CAD build for the part. Positions are in the model's coordinates, mm. A direction names the side the tool comes from. Coordinates: 2 decimals unless noted, no trailing zeros. Order: outer loops, then holes, each group sorted by start corner. A loop starts at its lowest first (then second) coordinate and runs counter-clockwise, first axis right, second up. Notation, with made-up numbers: M 43.25,23 L 91.25,23 A26 ccw 91.25,39 Z; hole C 48,-22.75 d10. An arc over 180 degrees is marked long. One line per item, written item: value.
Autodesk Inventor part; units mm, degrees
ref_plane "YZ Plane" through (0, 0, 0) normal (1, 0, 0) x (0, 1, 0)
ref_plane "XZ Plane" through (0, 0, 0) normal (0, 1, 0) x (-1, 0, 0)
ref_plane "XY Plane" through (0, 0, 0) normal (0, 0, 1) x (1, 0, 0)
sketch "Sketch1" plane through (0, 0, 0) normal (0, 0, 1) x (1, 0, 0)
  line L0 (0, 16.24) -> (0, -16.24) construction
  line L1 (-10, 0) -> (60, 0) construction
  line L2 (50, 11.6) -> (50, 9.6)
  line L3 (50, 9.6) -> (32, 9.6)
  line L4 (28, 11.6) -> (28, -9.6)
  line L5 (28, -9.6) -> (13, -9.6)
  line L6 (13, -9.6) -> (13, -11.6)
  line L7 (13, -11.6) -> (32, -11.6)
  line L8 (32, -11.6) -> (32, 9.6)
  line L9 (28, 11.6) -> (50, 11.6)
  point P0 (0, 0)
  dimension "d0" = 2
  dimension "d1" = 2
  dimension "d4" = 50
  dimension "d7" = 13
  dimension "d11" = 19.2
  dimension "d35" = 32
  dimension "d36" = 4
  dimension "d37" = 21.2
revolve "Revolution1" add sketch "Sketch1" angle 360 about axis through (0, 0, 0) along (0, -1, 0)
sketch "Sketch2" plane through (0, -9.6, 0) normal (0, -1, 0) x (1, 0, 0)
  line L0 (0, 70) -> (0, -70) construction
  line L1 (-70, 0) -> (70, 0) construction
  circle A0 centre (0, 0) radius 13 construction
  circle A1 centre (0, 0) radius 32 construction
  line L2 (15.5, -15.5) -> (-15.5, -15.5) construction
  line L3 (-15.5, -15.5) -> (-15.5, 15.5) construction
  line L4 (-15.5, 15.5) -> (15.5, 15.5) construction
  line L5 (15.5, 15.5) -> (15.5, -15.5) construction
  dimension "d14" = 31
  dimension "d15" = 31
hole "Hole1" at (15.5, -9.6, -15.5) at (-15.5, -9.6, -15.5) at (-15.5, -9.6, 15.5) at (15.5, -9.6, 15.5) direction (0, -1, 0) diameter 3.4 end through all countersink diameter 6.3 countersink angle 90
sketch "Sketch3" plane through (0, 11.6, 0) normal (0, 1, 0) x (1, 0, 0)
  line L0 (0, 70) -> (0, -70) construction
  line L1 (70, 0) -> (-70, 0) construction
  circle A0 centre (0, 0) radius 45 construction
  point P0 (0, 45)
  point P1 (-38.9711, 22.5)
  point P2 (-38.9711, -22.5)
  point P3 (0, -45)
  point P4 (38.9711, -22.5)
  point P5 (38.9711, 22.5)
  dimension "d23" = 90
  dimension "d26" = 360
hole "Hole2" at (0, 11.6, -45) at (-38.9711, 11.6, -22.5) at (-38.9711, 11.6, 22.5) at (0, 11.6, 45) at (38.9711, 11.6, 22.5) at (38.9711, 11.6, -22.5) direction (0, -1, 0) diameter 3.4 depth 2
fillet "Fillet1" radius 5 1 edges at (-32, 9.6, 0)
sketch "Sketch4" plane through (0, -9.6, 0) normal (0, 1, 0) x (1, 0, 0)
  line L0 (0, 70) -> (0, -70) construction
  line L1 (-70, 0) -> (70, 0) construction
  circle A0 centre (0, 16.6) radius 2
  circle A1 centre (12.5, -11) radius 2
  circle A2 centre (-12.5, -11) radius 2
  point P0 (0, 0)
  dimension "d39" = 4
  dimension "d54" = 16.6
  dimension "d55" = 4
  dimension "d56" = 25
  dimension "d57" = 11
extrude "Extrusion1" add sketch "Sketch4" along normal blind 4.75
sketch "Sketch5" plane through (0, -4.85, -16.6) normal (0, 1, 0) x (1, 0, 0)
  circle A0 centre (0, 0) radius 2 construction
  circle A1 centre (-12.5, -27.6) radius 2 construction
  circle A2 centre (12.5, -27.6) radius 2 construction
  circle A3 centre (12.5, -27.6) radius 2 construction
  point P0 (0, -16.6)
hole "Hole3" at (0, -4.85, -16.6) at (-12.5, -4.85, 11) at (12.5, -4.85, 11) direction (0, -1, 0) diameter 1.567 depth 6.3 tip angle 118
equation "\"d55\" = d39"
properties part number "Adapter_motor_planetarygearbox" material "Aluminum 6061"
Q1. Slice it at B-B (y = 7). List the corners of the cut face in (x, z).
Recorded:
outline: C 0,0 d65.23; hole C 0,0 d56
Q2. Slice it at A-A (z = 45). List the corners of the cut face in (x, y).
Recorded:
outline: M -21.79,9.6 L -1.7,9.6 L -1.7,11.6 L -21.79,11.6 Z; M 1.7,9.6 L 21.79,9.6 L 21.79,11.6 L 1.7,11.6 Z
Q3. Drill centre lines: line 1 along Z through (x, y) = (-15.5, -11.35); line 2 along Z through (x, y) = (0, 10.85); line 3 along Z through (x, y) = (0, -6.75). Where is each one in solid material? Low to high.
Recorded:
line 1: z = -28 to -17.2, -13.8 to 13.8, 17.2 to 28
line 2: z = -50 to -46.7, -43.3 to -28, 28 to 43.3, 46.7 to 50
line 3: z = -32 to -28, -18.6 to -17.38, -15.82 to -14.6, 28 to 32
Q4. Slice it at C-C (z = 23). Give the number of separate pieces and of enclosed holes in the cut face, plus the area to 3 significant figures.
Recorded:
separate pieces: 3
enclosed holes: 0
area: 446 mm^2
Q5. Mould opens along X. For faces 3 (the face through (-37.3, 9.6, -3.5)), 4 (the face through (-0.07, 10.59, -46.7)) say: released by +X, released by -X, zero draft, split by the parting line, or undercut.
Recorded:
face 3: zero draft
face 4: undercut
Q6. Pin check, flat tips, straight feed: pin 1 Ø2 at (y, z) = (-5, 5.5) entering from -X; pin 2 Ø4 at (x, z) = (-38.97, -22.5) entering from +Y; pin 3 Ø4 at (x, z) = (-38.97, 22.5) entering from -Y; pin 4 Ø2 at (x, z) = (12.5, 10) entering from +Y. Stop position of each tip, or through.
Recorded:
pin 1: stops at x = -31.68
pin 2: stops at y = 11.6
pin 3: stops at y = 9.6
pin 4: stops at y = -4.85
Q7. Which spindle directions (+Z, -Z, +X, -X, +Y, -Y) get a long thin tool onto all of the face, cutting with end or side? Do faces 1 (the face through (22, 11.6, -22)), 2 (the face through (12, -4.85, 12)). Say none if no direction does.
Recorded:
face 1: +Z, -Z, +X, -X, +Y
face 2: +Y
